The listing builds one solid part. Answer for the finished solid, in the listing's coordinates (mm). A direction names the side the tool comes from. Give positions to 0.01 mm unless a question says otherwise; leave off trailing zeros. Write each loop counter-clockwise with the first axis right and the second up, starting at its lowest first coordinate (ties: lowest second). Pieces come first, ordered by that corner, then holes. Notation, with made-up numbers: (15.5, -35.5) - (30.5, -35.5) arc R34 ccw to (30.5, 2.5) - close; hole circle Ø8 at (-15.75, -40). An arc over 180 degrees is marked (long way). Return JSON: item names as keys, results as strings.
from build123d import *

# Parameters (mm, degrees)
EXTRUDE_THIN1_DEPTH = 12
BOSS_EXTRUDE2_START = -12
BOSS_EXTRUDE2_DEPTH = 12


with BuildPart() as part:
    # Sketch1 → Extrude-Thin1 (new body)
    with BuildSketch(Plane.XY):
        with BuildLine():
            Line((5.107, -330.696), (5.107, -340.696))
            ThreePointArc((5.107, -340.696), (4.667660172, -341.756660172), (3.607, -342.196))
            Line((3.607, -342.196), (2.861, -342.196))
            ThreePointArc((2.861, -342.196), (0.383297839, -348.177702161), (6.365, -345.7))
            Line((6.365, -345.7), (6.365, 0))
            ThreePointArc((6.365, 0), (0, 6.365), (-6.365, 0))
            Line((-6.365, 0), (-6.365, -388))
            ThreePointArc((-6.365, -388), (0, -394.365), (6.365, -388))
            Line((6.365, -388), (6.365, -355.7))
            ThreePointArc((6.365, -355.7), (0.383297839, -353.222297839), (2.861, -359.204))
            Line((2.861, -359.204), (3.607, -359.204))
            ThreePointArc((3.607, -359.204), (4.667660172, -359.643339828), (5.107, -360.704))
            Line((5.107, -360.704), (5.107, -370.704))
            Line((5.107, -370.704), (4.591, -370.704))
            Line((4.591, -370.704), (4.591, -360.704))
            ThreePointArc((4.591, -360.704), (4.302793073, -360.008206927), (3.607, -359.72))
            Line((3.607, -359.72), (2.861, -359.72))
            ThreePointArc((2.861, -359.72), (0.01843074, -352.85743074), (6.881, -355.7))
            Line((6.881, -355.7), (6.881, -388))
            ThreePointArc((6.881, -388), (0, -394.881), (-6.881, -388))
            Line((-6.881, -388), (-6.881, 0))
            ThreePointArc((-6.881, 0), (0, 6.881), (6.881, 0))
            Line((6.881, 0), (6.881, -345.7))
            ThreePointArc((6.881, -345.7), (0.01843074, -348.54256926), (2.861, -341.68))
            Line((2.861, -341.68), (3.607, -341.68))
            ThreePointArc((3.607, -341.68), (4.302793073, -341.391793073), (4.591, -340.696))
            Line((4.591, -340.696), (4.591, -330.696))
            Line((4.591, -330.696), (5.107, -330.696))
        make_face()
    extrude(amount=EXTRUDE_THIN1_DEPTH)

    # Sketch3 → Boss-Extrude2 (add)
    with BuildSketch(Plane.XY.offset(12).offset(BOSS_EXTRUDE2_START)):
        with BuildLine():
            ThreePointArc((-5.361, -388), (0, -393.361), (5.361, -388))
            Line((5.361, -388), (5.361, -370.704))
            Line((5.361, -370.704), (5.107, -370.704))
            Line((5.107, -370.704), (5.107, -360.704))
            ThreePointArc((5.107, -360.704), (4.667660172, -359.643339828), (3.607, -359.204))
            Line((3.607, -359.204), (2.861, -359.204))
            ThreePointArc((2.861, -359.204), (0.383297839, -353.222297839), (6.365, -355.7))
            Line((6.365, -355.7), (6.365, -388))
            ThreePointArc((6.365, -388), (0, -394.365), (-6.365, -388))
            Line((-6.365, -388), (-6.365, 0))
            ThreePointArc((-6.365, 0), (0, 6.365), (6.365, 0))
            Line((6.365, 0), (6.365, -345.7))
            ThreePointArc((6.365, -345.7), (0.383297839, -348.177702161), (2.861, -342.196))
            Line((2.861, -342.196), (3.607, -342.196))
            ThreePointArc((3.607, -342.196), (4.667660172, -341.756660172), (5.107, -340.696))
            Line((5.107, -340.696), (5.107, -330.696))
            Line((5.107, -330.696), (5.361, -330.696))
            Line((5.361, -330.696), (5.361, 0))
            ThreePointArc((5.361, 0), (0, 5.361), (-5.361, 0))
            Line((-5.361, 0), (-5.361, -388))
        make_face()
        with BuildLine():
            ThreePointArc((5.361, -355.7), (1.093233047, -353.932233047), (2.861, -358.2))
            Line((2.861, -358.2), (3.607, -358.2))
            ThreePointArc((3.607, -358.2), (4.554437655, -358.386160944), (5.361, -358.916963347))
            Line((5.361, -358.916963347), (5.361, -355.7))
        make_face(mode=Mode.SUBTRACT)
        with BuildLine():
            ThreePointArc((2.861, -343.2), (1.093233047, -347.467766953), (5.361, -345.7))
            Line((5.361, -345.7), (5.361, -342.483036653))
            ThreePointArc((5.361, -342.483036653), (4.554437655, -343.013839056), (3.607, -343.2))
            Line((3.607, -343.2), (2.861, -343.2))
        make_face(mode=Mode.SUBTRACT)
    extrude(amount=BOSS_EXTRUDE2_DEPTH)


solid = part.part
Item 1: The mould has two halves that part along X. Classify faces 1 (the face through (5.361, -168, 6)), 2 (the face through (-6, -208, 12)), 3 (the face through (0.15, -394.88, 5.92)): +X half, -X half, draft (parallel to the pull), parting line (faces both ways), or undercut.
Answer below:
{"face 1": "undercut", "face 2": "draft", "face 3": "parting line"}
Item 2: A cutting plane is placed at B-B on z = 5.75. Determine the outline of the cut face in (x, y), then the cut area to 3 significant figures.
Answer below:
{"outline": "(-6.88, -388) arc R6.88 ccw to (6.88, -388) - (6.88, -355.7) arc R4.02 ccw (long way) to (2.86, -359.72) - (3.61, -359.72) arc R0.98 cw to (4.59, -360.7) - (4.59, -370.7) - (5.36, -370.7) - (5.36, -388) arc R5.36 cw to (-5.36, -388) - (-5.36, 0) arc R5.36 cw to (5.36, 0) - (5.36, -330.7) - (4.59, -330.7) - (4.59, -340.7) arc R0.98 cw to (3.61, -341.68) - (2.86, -341.68) arc R4.02 ccw (long way) to (6.88, -345.7) - (6.88, 0) arc R6.88 ccw to (-6.88, 0) - close; hole (2.86, -358.2) - (3.61, -358.2) arc R2.5 cw to (5.36, -358.92) - (5.36, -355.7) arc R2.5 ccw (long way) to start; hole (2.86, -343.2) arc R2.5 ccw (long way) to (5.36, -345.7) - (5.36, -342.48) arc R2.5 cw to (3.61, -343.2) - close", "area": "1,290 mm²"}
Item 3: For faces 4 (the face through (4.591, -336, 6)), 5 (the face through (6.881, -372, 6)), determine the directions among +Z, -Z, +X, -X, +Y, -Y from which every point of the face is accessible in a straight line to the end or side of a thin tool.
Answer below:
{"face 4": "+Z, -Z", "face 5": "+Z, -Z, +X, +Y, -Y"}
Item 4: A cutting plane is placed at A-A on y = -274.5. Determine the outline of the cut face in (x, z).
Answer below:
{"outline": "(-6.88, 0) - (-5.36, 0) - (-5.36, 12) - (-6.88, 12) - close; (5.36, 0) - (6.88, 0) - (6.88, 12) - (5.36, 12) - close"}
Item 5: Flat-ended cylindrical pins translate along their axes: P1, Ø0.6, axis at x = 3, z = 5, coming from the +Y side; P2, Ø0.8, axis at x = 5, z = 4, coming from the -Y side; P3, Ø1.5, axis at x = 2.5, z = 10, coming from the -Y side. Find the tip coordinate at first contact, or state that the pin passes through.
Answer below:
{"P1": "stops at y = 6.33", "P2": "stops at y = -393.12", "P3": "stops at y = -394.65"}
Item 6: Consider L1, parallel to X at y = -346, z = 6; L2, parallel to X at y = -345.7, z = 5; L3, parallel to X at y = -118, z = 1. Determine where each line is inside the solid, lowest interval first.
Answer below:
{"L1": "x = -6.88 to -5.36, -1.15 to 0.38, 5.34 to 6.87", "L2": "x = -6.88 to -5.36, -1.16 to 0.36, 5.36 to 6.88", "L3": "x = -6.88 to -5.36, 5.36 to 6.88"}
